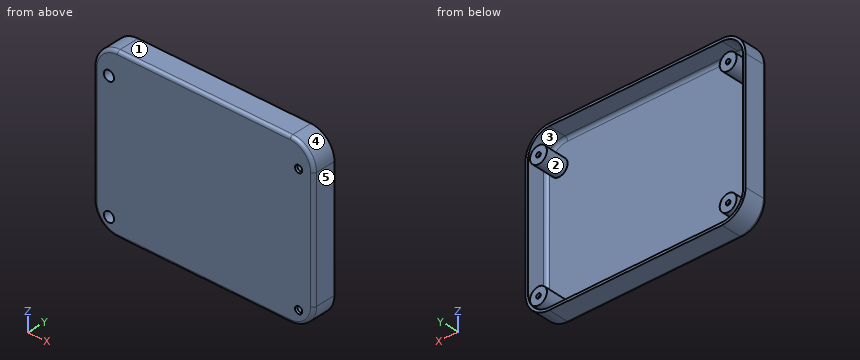
```python
from build123d import *

# Parameters (mm, degrees)
EXTRUDE_3_DEPTH     = 1.2
EXTRUDE_4_DEPTH     = 11
SKETCH_6_R          = 4
SKETCH_6_R_2        = 2.4
EXTRUDE_5_DEPTH     = 11
CUT_EXTRUDE_START   = -10
SKETCH_7_R          = 2.4
SKETCH_7_R_2        = 1.7
CUT_EXTRUDE_1_DEPTH = 10
EXTRUDE_START       = -1.2
SKETCH_8_R          = 2.4
SKETCH_8_R_2        = 1.1
EXTRUDE_6_DEPTH     = 1.2
FILLET_1_R          = 1.5


with BuildPart() as part:
    # 草图1 → 凸台-拉伸3 (new body)
    with BuildSketch(Plane(origin=(0, 0, 0), x_dir=(1, 0, 0), z_dir=(0, 1, 0))):
        with BuildLine():
            Line((51, -26), (51, 26))
            ThreePointArc((51, 26), (48.071067812, 33.071067812), (41, 36))
            Line((41, 36), (-41, 36))
            ThreePointArc((-41, 36), (-48.071067812, 33.071067812), (-51, 26))
            Line((-51, 26), (-51, -26))
            Line((-51, -26), (-51, -31))
            ThreePointArc((-51, -31), (-48.071067812, -38.071067812), (-41, -41))
            Line((-41, -41), (41, -41))
            ThreePointArc((41, -41), (48.071067812, -38.071067812), (51, -31))
            Line((51, -31), (51, -26))
        make_face()
    extrude(amount=EXTRUDE_3_DEPTH)

    # 草图4 → 凸台-拉伸4 (add)
    with BuildSketch(Plane(origin=(0, 0, 0), x_dir=(1, 0, 0), z_dir=(0, 1, 0))):
        with BuildLine():
            Line((-41, 37.2), (41, 37.2))
            ThreePointArc((41, 37.2), (48.919595949, 33.919595949), (52.2, 26))
            Line((52.2, 26), (52.2, -26))
            Line((52.2, -26), (52.2, -31))
            ThreePointArc((52.2, -31), (48.919633331, -38.919505702), (41.000127629, -42.199872371))
            Line((41.000127629, -42.199872371), (-41.000127629, -42.199872371))
            ThreePointArc((-41.000127629, -42.199872371), (-48.919633331, -38.919505702), (-52.2, -31))
            Line((-52.2, -31), (-52.2, -26))
            Line((-52.2, -26), (-52.2, 26))
            ThreePointArc((-52.2, 26), (-48.919595949, 33.919595949), (-41, 37.2))
        make_face()
        with BuildLine():
            Line((51, -26), (51, 26))
            ThreePointArc((51, 26), (48.071067812, 33.071067812), (41, 36))
            Line((41, 36), (-41, 36))
            ThreePointArc((-41, 36), (-48.071067812, 33.071067812), (-51, 26))
            Line((-51, 26), (-51, -26))
            Line((-51, -26), (-51, -31))
            ThreePointArc((-51, -31), (-48.071105194, -38.070977564), (-41.000127629, -40.999872371))
            Line((-41.000127629, -40.999872371), (41.000127629, -40.999872371))
            ThreePointArc((41.000127629, -40.999872371), (48.071105194, -38.070977564), (51, -31))
            Line((51, -31), (51, -26))
        make_face(mode=Mode.SUBTRACT)
    extrude(amount=EXTRUDE_4_DEPTH)

    # 草图6 → 凸台-拉伸5 (add)
    # profile 1 of 4: a face of its own
    with BuildSketch(Plane(origin=(0, 1.2, 0), x_dir=(1, 0, 0), z_dir=(0, 1, 0))):
        with Locations(Location((-45, 30, 0), (0, 0, 90))):
            Circle(SKETCH_6_R)
        with Locations(Location((-45, 30, 0), (0, 0, 270))):
            Circle(SKETCH_6_R_2, mode=Mode.SUBTRACT)
    # profile 2 of 4: a face of its own
    with BuildSketch(Plane(origin=(0, 1.2, 0), x_dir=(1, 0, 0), z_dir=(0, 1, 0))):
        with Locations(Location((45, 30, 0), (0, 0, 90))):
            Circle(SKETCH_6_R)
        with Locations(Location((45, 30, 0), (0, 0, 90))):
            Circle(SKETCH_6_R_2, mode=Mode.SUBTRACT)
    # profile 3 of 4: a face of its own
    with BuildSketch(Plane(origin=(0, 1.2, 0), x_dir=(1, 0, 0), z_dir=(0, 1, 0))):
        with Locations(Location((45, -30, 0), (0, 0, 90))):
            Circle(SKETCH_6_R)
        with Locations(Location((45, -30, 0), (0, 0, 270))):
            Circle(SKETCH_6_R_2, mode=Mode.SUBTRACT)
    # profile 4 of 4: a face of its own
    with BuildSketch(Plane(origin=(0, 1.2, 0), x_dir=(1, 0, 0), z_dir=(0, 1, 0))):
        with Locations(Location((-45, -30, 0), (0, 0, 90))):
            Circle(SKETCH_6_R)
        with Locations(Location((-45, -30, 0), (0, 0, 90))):
            Circle(SKETCH_6_R_2, mode=Mode.SUBTRACT)
    extrude(amount=EXTRUDE_5_DEPTH)

    # 草图7 → 切除-拉伸1 (cut)
    with BuildSketch(Plane(origin=(0, 1.2, 0), x_dir=(1, 0, 0), z_dir=(0, 1, 0)).offset(CUT_EXTRUDE_START)):
        with Locations(Location((-45, 30, 0), (0, 0, 90))):
            Circle(SKETCH_7_R)
        with Locations(Location((45, 30, 0), (0, 0, 270))):
            Circle(SKETCH_7_R_2)
        with Locations(Location((45, -30, 0), (0, 0, 270))):
            Circle(SKETCH_7_R_2)
        with Locations(Location((-45, -30, 0), (0, 0, 90))):
            Circle(SKETCH_7_R)
    extrude(amount=CUT_EXTRUDE_1_DEPTH, mode=Mode.SUBTRACT)

    # 草图8 → 凸台-拉伸6 (add)
    # profile 1 of 4: a face of its own
    with BuildSketch(Plane(origin=(0, 12.2, 0), x_dir=(1, 0, 0), z_dir=(0, 1, 0)).offset(EXTRUDE_START)):
        with Locations(Location((-45, 30, 0), (0, 0, 90))):
            Circle(SKETCH_8_R)
        with Locations(Location((-45, 30, 0), (0, 0, 270))):
            Circle(SKETCH_8_R_2, mode=Mode.SUBTRACT)
    # profile 2 of 4: a face of its own
    with BuildSketch(Plane(origin=(0, 12.2, 0), x_dir=(1, 0, 0), z_dir=(0, 1, 0)).offset(EXTRUDE_START)):
        with Locations(Location((45, 30, 0), (0, 0, 90))):
            Circle(SKETCH_8_R)
        with Locations(Location((45, 30, 0), (0, 0, 90))):
            Circle(SKETCH_8_R_2, mode=Mode.SUBTRACT)
    # profile 3 of 4: a face of its own
    with BuildSketch(Plane(origin=(0, 12.2, 0), x_dir=(1, 0, 0), z_dir=(0, 1, 0)).offset(EXTRUDE_START)):
        with Locations(Location((45, -30, 0), (0, 0, 270))):
            Circle(SKETCH_8_R)
        with Locations(Location((45, -30, 0), (0, 0, 270))):
            Circle(SKETCH_8_R_2, mode=Mode.SUBTRACT)
    # profile 4 of 4: a face of its own
    with BuildSketch(Plane(origin=(0, 12.2, 0), x_dir=(1, 0, 0), z_dir=(0, 1, 0)).offset(EXTRUDE_START)):
        with Locations(Location((-45, -30, 0), (0, 0, 90))):
            Circle(SKETCH_8_R)
        with Locations(Location((-45, -30, 0), (0, 0, 90))):
            Circle(SKETCH_8_R_2, mode=Mode.SUBTRACT)
    extrude(amount=EXTRUDE_6_DEPTH)

    # 圆角1
    # the kernel refuses this fillet: 1.5 mm, written as the material it adds along each edge
    with BuildSketch(Plane(origin=(-41, 1.2, -26), x_dir=(0, 0, -1), z_dir=(1, 0, 0))) as fillet_1_piece_1:
        with BuildLine():
            CenterArc((10 - FILLET_1_R, FILLET_1_R), FILLET_1_R, 270, 90)
            Line((10, FILLET_1_R), (10, 0))
            Line((10, 0), (10 - FILLET_1_R, 0))
        make_face()
    revolve(axis=Axis((-41, 1.2, -26), (0, 1, 0)), revolution_arc=90)
    with BuildSketch(Plane(origin=(-51, 1.2, 31), x_dir=(1, 0, 0), z_dir=(0, 0, -1)), Plane(origin=(51, 1.2, -26), x_dir=(-1, 0, 0), z_dir=(0, 0, 1))) as fillet_1_piece_2:
        with BuildLine():
            CenterArc((FILLET_1_R, -FILLET_1_R), FILLET_1_R, 90, 90)
            Line((0, -FILLET_1_R), (0, 0))
            Line((0, 0), (FILLET_1_R, 0))
        make_face()
    extrude(amount=57)
    with BuildSketch(Plane(origin=(41, 1.2, -26), x_dir=(1, 0, 0), z_dir=(0, 0, 1))) as fillet_1_piece_3:
        with BuildLine():
            CenterArc((10 - FILLET_1_R, FILLET_1_R), FILLET_1_R, 270, 90)
            Line((10, FILLET_1_R), (10, 0))
            Line((10, 0), (10 - FILLET_1_R, 0))
        make_face()
    revolve(axis=Axis((41, 1.2, -26), (0, 1, 0)), revolution_arc=90)
    with BuildSketch(Plane(origin=(-41.000127629, 1.2, 31), x_dir=(0, 0, 1), z_dir=(1, 0, 0))) as fillet_1_piece_4:
        with BuildLine():
            CenterArc((9.999872371 - FILLET_1_R, -FILLET_1_R), FILLET_1_R, 0, 90)
            Line((9.999872371, -FILLET_1_R), (9.999872371, 0))
            Line((9.999872371, 0), (9.999872371 - FILLET_1_R, 0))
        make_face()
    revolve(axis=Axis((-41.000127629, 1.2, 31), (0, -1, 0)), revolution_arc=90)
    with BuildSketch(Plane(origin=(41.000127629, 1.2, 40.999872371), x_dir=(0, 0, -1), z_dir=(-1, 0, 0))) as fillet_1_piece_5:
        with BuildLine():
            CenterArc((FILLET_1_R, -FILLET_1_R), FILLET_1_R, 90, 90)
            Line((0, -FILLET_1_R), (0, 0))
            Line((0, 0), (FILLET_1_R, 0))
        make_face()
    extrude(amount=82.000255259)
    with BuildSketch(Plane(origin=(41.000127629, 1.2, 31), x_dir=(1, 0, 0), z_dir=(0, 0, -1))) as fillet_1_piece_6:
        with BuildLine():
            CenterArc((9.999872371 - FILLET_1_R, -FILLET_1_R), FILLET_1_R, 0, 90)
            Line((9.999872371, -FILLET_1_R), (9.999872371, 0))
            Line((9.999872371, 0), (9.999872371 - FILLET_1_R, 0))
        make_face()
    revolve(axis=Axis((41.000127629, 1.2, 31), (0, -1, 0)), revolution_arc=90)
    with BuildSketch(Plane(origin=(41, 1.2, -36), x_dir=(0, 0, 1), z_dir=(-1, 0, 0))) as fillet_1_piece_7:
        with BuildLine():
            CenterArc((FILLET_1_R, FILLET_1_R), FILLET_1_R, 180, 90)
            Line((0, FILLET_1_R), (0, 0))
            Line((0, 0), (FILLET_1_R, 0))
        make_face()
    extrude(amount=82)
    # the kernel refuses this fillet: 1.5 mm, written as the material it takes off along each edge
    with BuildSketch(Plane(origin=(-41, 0, -26), x_dir=(-1, 0, 0), z_dir=(0, 0, 1))) as fillet_1_2_piece_1:
        with BuildLine():
            CenterArc((11.2 - FILLET_1_R, -FILLET_1_R), FILLET_1_R, 0, 90)
            Line((11.2, -FILLET_1_R), (11.2, 0))
            Line((11.2, 0), (11.2 - FILLET_1_R, 0))
        make_face()
    revolve(axis=Axis((-41, 0, -26), (0, -1, 0)), revolution_arc=90, mode=Mode.SUBTRACT)
    with BuildSketch(Plane(origin=(-52.2, 0, -26), x_dir=(1, 0, 0), z_dir=(0, 0, 1)), Plane(origin=(52.2, 0, 31), x_dir=(-1, 0, 0), z_dir=(0, 0, -1))) as fillet_1_2_piece_2:
        with BuildLine():
            CenterArc((FILLET_1_R, FILLET_1_R), FILLET_1_R, 180, 90)
            Line((0, FILLET_1_R), (0, 0))
            Line((0, 0), (FILLET_1_R, 0))
        make_face()
    extrude(amount=57, mode=Mode.SUBTRACT)
    with BuildSketch(Plane(origin=(-41.000127629, 0, 31), x_dir=(0, 0, 1), z_dir=(1, 0, 0))) as fillet_1_2_piece_3:
        with BuildLine():
            CenterArc((11.199872371 - FILLET_1_R, -FILLET_1_R), FILLET_1_R, 0, 90)
            Line((11.199872371, -FILLET_1_R), (11.199872371, 0))
            Line((11.199872371, 0), (11.199872371 - FILLET_1_R, 0))
        make_face()
    revolve(axis=Axis((-41.000127629, 0, 31), (0, -1, 0)), revolution_arc=90, mode=Mode.SUBTRACT)
    with BuildSketch(Plane(origin=(41.000127629, 0, 42.199872371), x_dir=(0, 0, -1), z_dir=(-1, 0, 0))) as fillet_1_2_piece_4:
        with BuildLine():
            CenterArc((FILLET_1_R, -FILLET_1_R), FILLET_1_R, 90, 90)
            Line((0, -FILLET_1_R), (0, 0))
            Line((0, 0), (FILLET_1_R, 0))
        make_face()
    extrude(amount=82.000255259, mode=Mode.SUBTRACT)
    with BuildSketch(Plane(origin=(41.000127629, 0, 31), x_dir=(1, 0, 0), z_dir=(0, 0, -1))) as fillet_1_2_piece_5:
        with BuildLine():
            CenterArc((11.199872371 - FILLET_1_R, -FILLET_1_R), FILLET_1_R, 0, 90)
            Line((11.199872371, -FILLET_1_R), (11.199872371, 0))
            Line((11.199872371, 0), (11.199872371 - FILLET_1_R, 0))
        make_face()
    revolve(axis=Axis((41.000127629, 0, 31), (0, -1, 0)), revolution_arc=90, mode=Mode.SUBTRACT)
    with BuildSketch(Plane(origin=(41, 0, -26), x_dir=(0, 0, -1), z_dir=(-1, 0, 0))) as fillet_1_2_piece_6:
        with BuildLine():
            CenterArc((11.2 - FILLET_1_R, -FILLET_1_R), FILLET_1_R, 0, 90)
            Line((11.2, -FILLET_1_R), (11.2, 0))
            Line((11.2, 0), (11.2 - FILLET_1_R, 0))
        make_face()
    revolve(axis=Axis((41, 0, -26), (0, -1, 0)), revolution_arc=90, mode=Mode.SUBTRACT)
    with BuildSketch(Plane(origin=(-41, 0, -37.2), x_dir=(0, 0, 1), z_dir=(1, 0, 0))) as fillet_1_2_piece_7:
        with BuildLine():
            CenterArc((FILLET_1_R, -FILLET_1_R), FILLET_1_R, 90, 90)
            Line((0, -FILLET_1_R), (0, 0))
            Line((0, 0), (FILLET_1_R, 0))
        make_face()
    extrude(amount=82, mode=Mode.SUBTRACT)


solid = part.part
```
Geometry check sheet. Reference: the model listing, model coordinates, mm. Face numbers are marked on the shaded views. A direction names the side the tool comes from. Give positions to 0.01 mm unless a question says otherwise; leave off trailing zeros. Write each loop counter-clockwise with the first axis right and the second up, starting at its lowest first coordinate (ties: lowest second). Pieces come first, ordered by that corner, then holes.
1) Access from +Z, -Z, +X, -X, +Y, -Y to the whole of each face (thin tool, end or side, straight path). Record for the marked faces 1 and 2.
2) Section check C-C, the plane z = 5.5. Record the boundary of the cut face in (x, y), and give its area (3 significant figures).
3) Release check for a two-part mould opening along Z. For the marked faces 3, 4 and 5 record: pulls with the +Z half, pulls with the -Z half, needs draft (parallel to the pull), parting line crosses it, or undercut.
4) Material ranges on L1, parallel to X at y = 11.75, z = 30; L2, parallel to X at y = 7.5, z = 30; L3, parallel to X at y = 9.25, z = -6, recorded low to high.
5) Gauge pin test, flat ends, axial feed: pin 1 (2.5 mm diameter, centred on x = -45, z = 30, fed in from +Y); pin 2 (4.5 mm diameter, centred on x = -45, z = -30, fed in from -Y); pin 3 (6 mm diameter, centred on x = 15.5, z = -4.5, fed in from +Y). Record the tip position at first contact, or that the pin passes through.
6) Section check A-A, the plane y = 7. State how many separate pieces and enclosed holes the cut face has, and give its area (3 significant figures).
7) Section check B-B, the plane x = -38.5. Record the boundary of the cut face in (y, z).
Computed:
1. face 1: +Z, +X, -X, +Y, -Y
1. face 2: +Y
2. outline: (-52.2, 1.5) arc R1.5 ccw to (-50.7, 0) - (50.7, 0) arc R1.5 ccw to (52.2, 1.5) - (52.2, 11) - (51, 11) - (51, 2.7) arc R1.5 cw to (49.5, 1.2) - (-49.5, 1.2) arc R1.5 cw to (-51, 2.7) - (-51, 11) - (-52.2, 11) - close
2. area: 149 mm2
3. face 3: undercut
3. face 4: pulls with the +Z half
3. face 5: needs draft
4. L1: x = -49 to -46.1, -43.9 to -41, 41 to 43.9, 46.1 to 49
4. L2: x = -52.2 to -51, -49 to -47.4, -42.6 to -41, 41 to 42.6, 47.4 to 49, 51 to 52.2
4. L3: x = -52.2 to -51, 51 to 52.2
5. pin 1: stops at y = 12.2
5. pin 2: stops at y = 11
5. pin 3: stops at y = 1.2
6. separate pieces: 5
6. enclosed holes: 5
6. area: 542 mm2
7. outline: (0, -35.7) arc R1.5 ccw to (1.5, -37.2) - (11, -37.2) - (11, -36) - (2.7, -36) arc R1.5 cw to (1.2, -34.5) - (1.2, 39.5) arc R1.5 cw to (2.7, 41) - (11, 41) - (11, 42.2) - (1.5, 42.2) arc R1.5 ccw to (0, 40.7) - close
